from build123d import *

# Parameters (mm, degrees)
SKETCH_1_W          = 8
SKETCH_1_H          = 8
EXTRUDE_1_DEPTH     = 10
SKETCH_2_R          = 2.5
CUT_EXTRUDE_1_DEPTH = 16.099668871
SKETCH_4_R          = 2.5
CUT_EXTRUDE_2_DEPTH = 16.099668871
FILLET_1_R          = 1


with BuildPart() as part:
    # 草图1 → 凸台-拉伸1 (new body)
    with BuildSketch(Plane.XY):
        with Locations((4, 4)):
            Rectangle(SKETCH_1_W, SKETCH_1_H)
    extrude(amount=EXTRUDE_1_DEPTH)

    # 草图2 → 切除-拉伸1 (cut, through all)
    with BuildSketch(Plane.XY.offset(10)):
        with Locations((4, 3)):
            Circle(SKETCH_2_R)
    extrude(amount=-CUT_EXTRUDE_1_DEPTH, mode=Mode.SUBTRACT)

    # 草图4 → 切除-拉伸2 (cut, through all)
    with BuildSketch(Plane(origin=(8, 0, 0), x_dir=(0, 0, -1), z_dir=(1, 0, 0))):
        with Locations((-5, 4)):
            Circle(SKETCH_4_R)
    extrude(amount=-CUT_EXTRUDE_2_DEPTH, mode=Mode.SUBTRACT)

    # 圆角1
    # the kernel refuses this fillet: 1 mm, written as the material it takes off along each edge
    with BuildSketch(Plane(origin=(7, 7, 9), x_dir=(1, 0, 0), z_dir=(0, 1, 0))) as fillet_1_piece_1_section:
        Polygon((0, 0), (FILLET_1_R, 0), (FILLET_1_R, -FILLET_1_R), (0, -FILLET_1_R), align=None)
    fillet_1_piece_1 = extrude(amount=FILLET_1_R, mode=Mode.PRIVATE)
    fillet_1_piece_1 = fillet_1_piece_1 - Plane(origin=(7, 7, 9), x_dir=(-0.7071067811865475, 0, -0.7071067811865475), z_dir=(0, 1, 0)) * Sphere(FILLET_1_R, mode=Mode.PRIVATE)
    add(fillet_1_piece_1, mode=Mode.SUBTRACT)
    with BuildSketch(Plane(origin=(7, 1, 9), x_dir=(0, 0, 1), z_dir=(1, 0, 0))) as fillet_1_piece_2_section:
        Polygon((0, 0), (FILLET_1_R, 0), (FILLET_1_R, FILLET_1_R), (0, FILLET_1_R), align=None)
    fillet_1_piece_2 = extrude(amount=FILLET_1_R, mode=Mode.PRIVATE)
    fillet_1_piece_2 = fillet_1_piece_2 - Plane(origin=(7, 1, 9), x_dir=(0, 0.7071067811865475, -0.7071067811865475), z_dir=(1, 0, 0)) * Sphere(FILLET_1_R, mode=Mode.PRIVATE)
    add(fillet_1_piece_2, mode=Mode.SUBTRACT)
    with BuildSketch(Plane(origin=(1, 7, 9), x_dir=(-1, 0, 0), z_dir=(0, 1, 0))) as fillet_1_piece_3_section:
        Polygon((0, 0), (FILLET_1_R, 0), (FILLET_1_R, FILLET_1_R), (0, FILLET_1_R), align=None)
    fillet_1_piece_3 = extrude(amount=FILLET_1_R, mode=Mode.PRIVATE)
    fillet_1_piece_3 = fillet_1_piece_3 - Plane(origin=(1, 7, 9), x_dir=(0.7071067811865475, 0, -0.7071067811865475), z_dir=(0, 1, 0)) * Sphere(FILLET_1_R, mode=Mode.PRIVATE)
    add(fillet_1_piece_3, mode=Mode.SUBTRACT)
    with BuildSketch(Plane(origin=(1, 1, 9), x_dir=(0, 0, 1), z_dir=(-1, 0, 0))) as fillet_1_piece_4_section:
        Polygon((0, 0), (FILLET_1_R, 0), (FILLET_1_R, -FILLET_1_R), (0, -FILLET_1_R), align=None)
    fillet_1_piece_4 = extrude(amount=FILLET_1_R, mode=Mode.PRIVATE)
    fillet_1_piece_4 = fillet_1_piece_4 - Plane(origin=(1, 1, 9), x_dir=(0, 0.7071067811865475, -0.7071067811865475), z_dir=(-1, 0, 0)) * Sphere(FILLET_1_R, mode=Mode.PRIVATE)
    add(fillet_1_piece_4, mode=Mode.SUBTRACT)
    with BuildSketch(Plane(origin=(1, 7, 1), x_dir=(-1, 0, 0), z_dir=(0, 1, 0))) as fillet_1_piece_5_section:
        Polygon((0, 0), (FILLET_1_R, 0), (FILLET_1_R, -FILLET_1_R), (0, -FILLET_1_R), align=None)
    fillet_1_piece_5 = extrude(amount=FILLET_1_R, mode=Mode.PRIVATE)
    fillet_1_piece_5 = fillet_1_piece_5 - Plane(origin=(1, 7, 1), x_dir=(0.7071067811865475, 0, 0.7071067811865475), z_dir=(0, 1, 0)) * Sphere(FILLET_1_R, mode=Mode.PRIVATE)
    add(fillet_1_piece_5, mode=Mode.SUBTRACT)
    with BuildSketch(Plane(origin=(7, 7, 1), x_dir=(1, 0, 0), z_dir=(0, 1, 0))) as fillet_1_piece_6_section:
        Polygon((0, 0), (FILLET_1_R, 0), (FILLET_1_R, FILLET_1_R), (0, FILLET_1_R), align=None)
    fillet_1_piece_6 = extrude(amount=FILLET_1_R, mode=Mode.PRIVATE)
    fillet_1_piece_6 = fillet_1_piece_6 - Plane(origin=(7, 7, 1), x_dir=(-0.7071067811865475, 0, 0.7071067811865475), z_dir=(0, 1, 0)) * Sphere(FILLET_1_R, mode=Mode.PRIVATE)
    add(fillet_1_piece_6, mode=Mode.SUBTRACT)
    with BuildSketch(Plane(origin=(7, 1, 1), x_dir=(0, 0, -1), z_dir=(1, 0, 0))) as fillet_1_piece_7_section:
        Polygon((0, 0), (FILLET_1_R, 0), (FILLET_1_R, -FILLET_1_R), (0, -FILLET_1_R), align=None)
    fillet_1_piece_7 = extrude(amount=FILLET_1_R, mode=Mode.PRIVATE)
    fillet_1_piece_7 = fillet_1_piece_7 - Plane(origin=(7, 1, 1), x_dir=(0, 0.7071067811865475, 0.7071067811865475), z_dir=(1, 0, 0)) * Sphere(FILLET_1_R, mode=Mode.PRIVATE)
    add(fillet_1_piece_7, mode=Mode.SUBTRACT)
    with BuildSketch(Plane(origin=(1, 1, 1), x_dir=(0, 0, -1), z_dir=(-1, 0, 0))) as fillet_1_piece_8_section:
        Polygon((0, 0), (FILLET_1_R, 0), (FILLET_1_R, FILLET_1_R), (0, FILLET_1_R), align=None)
    fillet_1_piece_8 = extrude(amount=FILLET_1_R, mode=Mode.PRIVATE)
    fillet_1_piece_8 = fillet_1_piece_8 - Plane(origin=(1, 1, 1), x_dir=(0, 0.7071067811865475, 0.7071067811865475), z_dir=(-1, 0, 0)) * Sphere(FILLET_1_R, mode=Mode.PRIVATE)
    add(fillet_1_piece_8, mode=Mode.SUBTRACT)
    with BuildSketch(Plane(origin=(8, 7, 10), x_dir=(0, 0, -1), z_dir=(0, -1, 0)), Plane(origin=(1, 8, 10), x_dir=(0, 0, -1), z_dir=(1, 0, 0)), Plane(origin=(0, 1, 10), x_dir=(0, 0, -1), z_dir=(0, 1, 0)), Plane(origin=(7, 0, 0), x_dir=(0, 1, 0), z_dir=(-1, 0, 0))) as fillet_1_piece_9:
        with BuildLine():
            CenterArc((FILLET_1_R, -FILLET_1_R), FILLET_1_R, 90, 90)
            Line((0, -FILLET_1_R), (0, 0))
            Line((0, 0), (FILLET_1_R, 0))
        make_face()
    extrude(amount=6, mode=Mode.SUBTRACT)
    with BuildSketch(Plane(origin=(1, 8, 0), x_dir=(0, 0, 1), z_dir=(1, 0, 0)), Plane(origin=(8, 7, 0), x_dir=(0, 0, 1), z_dir=(0, -1, 0)), Plane(origin=(0, 1, 0), x_dir=(0, 0, 1), z_dir=(0, 1, 0)), Plane(origin=(7, 0, 10), x_dir=(0, 1, 0), z_dir=(-1, 0, 0))) as fillet_1_piece_10:
        with BuildLine():
            CenterArc((FILLET_1_R, FILLET_1_R), FILLET_1_R, 180, 90)
            Line((0, FILLET_1_R), (0, 0))
            Line((0, 0), (FILLET_1_R, 0))
        make_face()
    extrude(amount=6, mode=Mode.SUBTRACT)
    with BuildSketch(Plane(origin=(0, 8, 1), x_dir=(1, 0, 0), z_dir=(0, 0, 1)), Plane(origin=(0, 0, 1), x_dir=(0, 1, 0), z_dir=(0, 0, 1))) as fillet_1_piece_11:
        with BuildLine():
            CenterArc((FILLET_1_R, -FILLET_1_R), FILLET_1_R, 90, 90)
            Line((0, -FILLET_1_R), (0, 0))
            Line((0, 0), (FILLET_1_R, 0))
        make_face()
    extrude(amount=8, mode=Mode.SUBTRACT)
    with BuildSketch(Plane(origin=(8, 8, 1), x_dir=(-1, 0, 0), z_dir=(0, 0, 1)), Plane(origin=(8, 0, 1), x_dir=(0, 1, 0), z_dir=(0, 0, 1))) as fillet_1_piece_12:
        with BuildLine():
            CenterArc((FILLET_1_R, FILLET_1_R), FILLET_1_R, 180, 90)
            Line((0, FILLET_1_R), (0, 0))
            Line((0, 0), (FILLET_1_R, 0))
        make_face()
    extrude(amount=8, mode=Mode.SUBTRACT)


solid = part.part
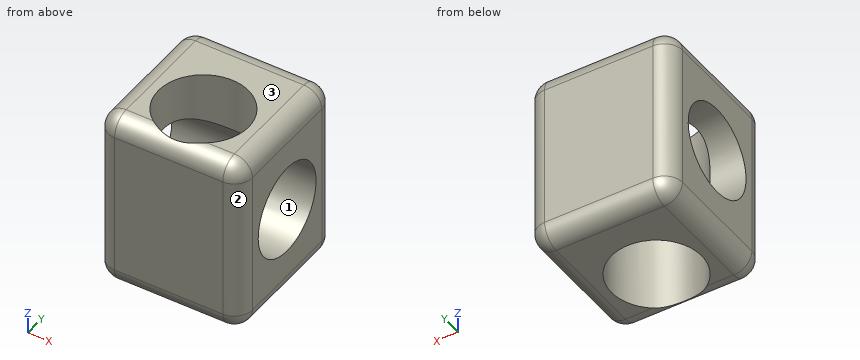
The model under review builds one solid part; all positions refer to its coordinate system, in mm. Face numbers are marked on the shaded views. Give positions to 0.01 mm unless a question says otherwise; leave off trailing zeros. Order: outer loops, then holes, each group sorted by start corner. A loop starts at its lowest first (then second) coordinate and runs counter-clockwise, first axis right, second up. Notation, with made-up numbers: M 83,60 L 115,60 A15 cw 115,72 Z; hole C 39.5,85.25 d10. An arc over 180 degrees is marked long. One line per question, with ' | ' between items. Start each with the question number.
1) Consider section D-D, the plane z = 1.75. Give the boundary of the cut face in (x, y), then the cut area to 3 significant figures.
2) Wall thickness on L1, parallel to Y at x = 4, z = 7.75; L2, parallel to Y at x = 5.5, z = 5; L3, parallel to Z at x = 7.25, y = 5: over which ranges is each line inside the solid? List them lowest first. Write a range as from..to.
3) Mouldability with a two-part tool opening along Z and no side actions: class the marked faces 1, 2 and 3 as pulls with the +Z half, pulls with the -Z half, needs draft (parallel to the pull), parting line crosses it, or undercut.
4) Consider section C-C, the plane x = 4. Give the boundary of the cut face in (y, z), then the cut area to 3 significant figures.
5) Clearance check with a flat-ended pin moving along its axis: P1, Ø2, axis at x = 3.5, y = 2.5, coming from the -Z side. State where the tip first meets the part, or that it passes through.
6) Consider section B-B, the plane y = 2.25. Give the boundary of the cut face in (x, z).
7) Consider section A-A, the plane z = 5. Give the boundary of the cut face in (x, y), then the cut area to 3 significant figures.
Found:
1) outline: M 0,1 A1 ccw 1,0 L 7,0 A1 ccw 8,1 L 8,7 A1 ccw 7,8 L 1,8 A1 ccw 0,7 Z; hole C 4,3 d5 | area: 43.5 mm²
2) L1: y = 0..0.5, 5.5..8 | L2: y = 0..1, 6.5..8 | L3: z = 0.03..2.71, 7.29..9.97
3) face 1: undercut | face 2: needs draft | face 3: pulls with the +Z half
4) outline: M 0,1 A1 ccw 0.5,0.13 L 0.5,9.87 A1 ccw 0,9 Z; M 5.5,0 L 7,0 A1 ccw 8,1 L 8,9 A1 ccw 7,10 L 5.5,10 L 5.5,7 A2.5 cw 5.5,3 Z | area: 26.4 mm²
5) P1: passes through
6) outline: M 0,1 A1 ccw 1,0 L 1.62,0 L 1.62,3.21 L 0,3.21 Z; M 0,6.79 L 1.62,6.79 L 1.62,10 L 1,10 A1 ccw 0,9 Z; M 6.38,0 L 7,0 A1 ccw 8,1 L 8,3.21 L 6.38,3.21 Z; M 6.38,6.79 L 8,6.79 L 8,9 A1 ccw 7,10 L 6.38,10 Z
7) outline: M 0,1 A1 ccw 1,0 L 7,0 A1 ccw 8,1 L 8,1.5 L 6,1.5 A2.5 cw 2,1.5 L 0,1.5 Z; M 0,6.5 L 8,6.5 L 8,7 A1 ccw 7,8 L 1,8 A1 ccw 0,7 Z | area: 20.3 mm²
